```python
from build123d import *

# Parameters (mm, degrees)
F0_W     = 354
F0_H     = 138.5
F1_DEPTH = 1.5
F2_R     = 3
F3_DEPTH = 12.5


with BuildPart() as f1:
    # F0 (on Front) → F1 (new body, symmetric)
    with BuildSketch(Plane.XZ):
        Rectangle(F0_W, F0_H)
    extrude(amount=F1_DEPTH, both=True)

    # F2 (on Front) → F3 (cut, symmetric)
    with BuildSketch(Plane.XZ):
        with Locations((-165, 57.25)):
            Circle(F2_R)
        with Locations((-165, -57.25)):
            Circle(F2_R)
        with Locations((165, 57.25)):
            Circle(F2_R)
        with Locations((165, -57.25)):
            Circle(F2_R)
    extrude(amount=F3_DEPTH, both=True, mode=Mode.SUBTRACT)


solid = f1.part
```
Model file for the job. Use its own axes, mm. Coordinates: 2 decimals unless noted, no trailing zeros. Use CSV: the item, a comma, the result in double quotes. Start each with the question number.
1. Probe probe 1 along Z at (x, y) = (165, 0.8); probe 2 along X at (y, z) = (-0.05, 57.25); probe 3 along X at (y, z) = (0.95, 55.5). List the from-to ranges inside material, lowest first. Write a range as [from, to].
2. Flat gauge pins, fed straight in: pin 1 (7 mm diameter, centred on x = -165, z = 57.25, fed in from -Y); pin 2 (3.5 mm diameter, centred on x = 165, z = 57.25, fed in from +Y). Where does each tip first touch, or does it go through?
3. Two-plate mould, pull along Z, no slides. Class faces 1 (the cylindrical face through (-163.39, -0.02, 59.78)), 2 (the flat face through (-2, 1.5, 1)): pulls with the +Z half, pulls with the -Z half, needs draft (parallel to the pull), parting line crosses it, or undercut.
Entries:
1,probe 1,"z = [-69.25, -60.25], [-54.25, 54.25], [60.25, 69.25]"
1,probe 2,"x = [-177, -168], [-162, 162], [168, 177]"
1,probe 3,"x = [-177, -167.44], [-162.56, 162.56], [167.44, 177]"
2,pin 1,"stops at y = -1.5"
2,pin 2,"passes through"
3,face 1,"undercut"
3,face 2,"needs draft"
